from build123d import *

# Parameters (mm, degrees)
F1_DEPTH        = 5
F2_W            = 10
F2_H            = 10
F3_DEPTH        = 4
F5_D            = 4
F5_CBORE_D      = 6.5
F5_CBORE_DEPTH  = 2
F7_DEPTH        = 4
F9_D            = 4
F10_R           = 2
F11_DEPTH       = 2
F12_R           = 4.99999
F14_D           = 4
F14_CBORE_D     = 7
F14_CBORE_DEPTH = 1.5


# Not quite as in the source:
# - a fillet or chamfer is up to 0.001 mm smaller than in the source, because OpenCascade refuses the exact size


with BuildPart() as f1:
    # F0 (on Top) → F1 (new body)
    with BuildSketch(Plane.XY):
        Polygon((16.5, -25), (16.5, 25), (12.5, 25), (12.5, -5), (-12.5, -5), (-12.5, 25), (-16.5, 25), (-16.5, -25), align=None)
    extrude(amount=F1_DEPTH)

    # F2 (on face) → F3 (join)
    with BuildSketch(Plane(origin=(-16.5, 0, 0), x_dir=(0, -1, 0), z_dir=(-1, 0, 0))):
        with Locations((-20, 5)):
            Rectangle(F2_W, F2_H)
    extrude(amount=-F3_DEPTH)

    # F5 (through all)
    with Locations(Plane(origin=(-16.5, 0, 0), x_dir=(0, -1, 0), z_dir=(-1, 0, 0))):
        with Locations((-20, 5)):
            CounterBoreHole(F5_D / 2, F5_CBORE_D / 2, F5_CBORE_DEPTH)

    # F6 (on face) → F7 (join)
    with BuildSketch(Plane.YZ.offset(16.5)):
        with BuildLine():
            Line((22, 5), (25, 5))
            Line((25, 5), (25, 10))
            Line((25, 10), (15, 10))
            Line((15, 10), (15, 5))
            Line((15, 5), (18, 5))
            ThreePointArc((18, 5), (20, 3), (22, 5))
        make_face()
    extrude(amount=-F7_DEPTH)

    # F9 (through all)
    with Locations(Plane.YZ.offset(16.5)):
        with Locations((20, 5)):
            Hole(F9_D / 2)

    # F10 (on face) → F11 (cut)
    with BuildSketch(Plane.YZ.offset(16.5)):
        Polygon((20.9512871128, 1.8797618421), (23.1778490671, 4.263719727), (22.2265619542, 7.383957885), (19.0487128872, 8.1202381579), (16.8221509329, 5.736280273), (17.7734380458, 2.616042115), align=None)
        with Locations((20, 5)):
            Circle(F10_R, mode=Mode.SUBTRACT)
    extrude(amount=-F11_DEPTH, mode=Mode.SUBTRACT)

    # F12 (radius 5 in the source; OpenCascade refuses exactly that, so slightly less here)
    f12_edges = [f1.edges().sort_by_distance(p)[0] for p in [
        (14.5, 25, 10),
        (14.5, 15, 10),
        (-14.5, 15, 10),
        (-14.5, 25, 10),
        (0, -25, 5),
        (0, -5, 5),
    ]]
    fillet(f12_edges, radius=F12_R)

    # F14 (through all)
    with Locations(Plane.XY.offset(5)):
        with Locations((-8.25, -15.0438509881), (8.25, -15.0438509881)):
            CounterBoreHole(F14_D / 2, F14_CBORE_D / 2, F14_CBORE_DEPTH)


solid = f1.part
Here's how the part is built. I have some questions about the finished solid (model axes, mm). A direction names the side the tool comes from. Give positions to 0.01 mm unless a question says otherwise; leave off trailing zeros. Write each loop counter-clockwise with the first axis right and the second up, starting at its lowest first coordinate (ties: lowest second). Pieces come first, ordered by that corner, then holes. Notation, with made-up numbers: (-23, 23.5) -> (22, 23.5) arc R10 ccw to (22, 38.5) -> close; hole circle Ø5 at (-8, 2). An arc over 180 degrees is marked (long way). Use one line per item in the form item = value. Start each with the question number.
1. If I drill on L1, parallel to Z at x = 13, y = 20; L2, parallel to X at y = 22, z = 7.5; L3, parallel to X at y = 4.5, z = 4.75, over which ranges is the centre line in solid material (lowest first)?
2. On a 3-axis mill with a long thin cutter (end or side, diameter ignored), from which of +Z, -Z, +X, -X, +Y, -Y can I reach the whole of each face in a straight line? I mean faces 4 (the face through (15.51, 22.71, 5.8)), 5 (the face through (-15.514, 23.247, 5.143)), 6 (the face through (10, -17, 3.5)), 7 (the face through (-14, 24, 8)). Say none if no direction works.
3. Imagine slicing it at B-B on y = 7.5. List the corners of the cut face in (x, z) for me, plus the area to 3 significant figures.
4. Thinking about a two-plate mould opening in X: for faces 1 (the face through (0, -6, 3)), 2 (the face through (-14, 25, 2)), 3 (the face through (-16.5, 0, 3)), which applies, +X half, -X half, draft (parallel to the pull), parting line (faces both ways), or undercut?
5. Will these pins go through, and if not, where does the flat tip stop? pin 1 Ø6 at (y, z) = (12.5, 6.5) entering from +X; pin 2 Ø5 at (x, z) = (-7, 6) entering from +Y; pin 3 Ø7.5 at (x, y) = (8.5, -14.5) entering from +Z; pin 4 Ø3 at (y, z) = (20.5, 6) entering from -X.
Entries:
q1.L1 = 0 to 3, 7 to 10
q1.L2 = -14.5 to -12.5, 12.5 to 16.5
q1.L3 = -16.5 to -12.5, 12.5 to 16.5
q2.face_4 = +X
q2.face_5 = -X
q2.face_6 = +Z
q2.face_7 = +Z, +X, -X, +Y
q3.outline = (-16.5, 0) -> (-12.5, 0) -> (-12.5, 5) -> (-16.5, 5) -> close; (12.5, 0) -> (16.5, 0) -> (16.5, 5) -> (12.5, 5) -> close
q3.area = 40.0 mm²
q4.face_1 = undercut
q4.face_2 = draft
q4.face_3 = -X half
q5.pin_1 = 16.5
q5.pin_2 = -6.43
q5.pin_3 = 5
q5.pin_4 = -14.5
